Build history of the part. All positions in model axes, mm. A direction names the side the tool comes from. Round coordinates to 2 decimals unless told otherwise and drop trailing zeros. Write each loop counter-clockwise with the first axis right and the second up, starting at its lowest first coordinate (ties: lowest second). Pieces come first, ordered by that corner, then holes. Notation, with made-up numbers: (-24.5, 21.25) - (-7.5, 21.25) arc R6 cw to (-7.5, 30.25) - close; hole circle Ø4 at (84.25, -16.5). An arc over 180 degrees is marked (long way). One line per question, with ' | ' between items.
from build123d import *

# Parameters (mm, degrees)
F1_DEPTH = 50.8
F3_DEPTH = 25.4
F5_DEPTH = 12.7
F6_DEPTH = 12.7
F8_DEPTH = 25.401
F4_R     = 12.7
F9_DEPTH = 25.401


with BuildPart() as f1:
    # F0 (on Front) → F1 (new body)
    with BuildSketch(Plane.XZ):
        Polygon((-36.9852854972, 36.8870242119), (-62.3852854972, 36.8870242119), (-62.3852854972, -64.7129757881), (64.6147145028, -64.7129757881), (64.6147145028, -39.3129757881), (-36.9852854972, -39.3129757881), align=None)
    extrude(amount=F1_DEPTH)

    # F2 (on face) → F3 (cut)
    with BuildSketch(Plane.XY.offset(-39.3129757881)):
        with BuildLine():
            ThreePointArc((64.6147145028, -25.4), (57.1752267449, -43.3605122421), (39.2147145028, -50.8))
            Line((39.2147145028, -50.8), (64.6147145028, -50.8))
            Line((64.6147145028, -50.8), (64.6147145028, -25.4))
        make_face()
        with BuildLine():
            ThreePointArc((39.2147145028, 0), (57.1752267449, -7.4394877579), (64.6147145028, -25.4))
            Line((64.6147145028, -25.4), (64.6147145028, 0))
            Line((64.6147145028, 0), (39.2147145028, 0))
        make_face()
    extrude(amount=-F3_DEPTH, mode=Mode.SUBTRACT)

    # F5 (add): a face of the model
    f5_faces = [f1.faces().sort_by_distance(p)[0] for p in [
        (-36.9852854972, -25.4, -1.2129757881),
    ]]
    extrude(f5_faces, amount=F5_DEPTH)

    # F6 (cut): a face of the model
    f6_faces = [f1.faces().sort_by_distance(p)[0] for p in [
        (-62.3852854972, -25.4, -13.9129757881),
    ]]
    extrude(f6_faces, amount=-F6_DEPTH, mode=Mode.SUBTRACT)

    # F7 (on face) → F8 (cut, through all)
    with BuildSketch(Plane.YZ.offset(-24.2852854972)):
        with BuildLine():
            Line((-38.1, 36.8870242119), (-38.1, 11.4870242119))
            ThreePointArc((-38.1, 11.4870242119), (-25.4, -1.2129757881), (-12.7, 11.4870242119))
            Line((-12.7, 11.4870242119), (-12.7, 36.8870242119))
            Line((-12.7, 36.8870242119), (-38.1, 36.8870242119))
        make_face()
    extrude(amount=-F8_DEPTH, mode=Mode.SUBTRACT)

    # F4 (on face) → F9 (cut, through all)
    with BuildSketch(Plane.XY.offset(-39.3129757881)):
        with Locations((1.1147145028, -25.4)):
            Circle(F4_R)
        with Locations((39.2147145028, -25.4)):
            Circle(F4_R)
    extrude(amount=-F9_DEPTH, mode=Mode.SUBTRACT)


solid = f1.part
Q1. Pull direction Y, two halves, no side cores. Call faces 1 (the cylindrical face through (-36.81, -25.68, -1.21)), 2 (the flat face through (21, -25, -39.313)), 3 (the flat face through (-26, 0, -26)), 4 (the flat face through (-26, -50.8, -26)): +Y half, -Y half, draft (parallel to the pull), parting line (faces both ways), or undercut.
Found:
face 1: undercut | face 2: draft | face 3: +Y half | face 4: -Y half
Q2. Drill centre lines: L1, parallel to Y at x = -32, z = 12.5; L2, parallel to Z at x = -8.5, y = -9.5; L3, parallel to X at y = -7, z = 28.5. Where is each one in solid material? Low to high. Write a range as from..to.
Found:
L1: -50.8..-38.1, -12.7..0 | L2: -64.71..-39.31 | L3: -49.69..-24.29
Q3. Saw through at C-C, the plane z = -56.5. List the corners of the cut face in (x, y), then the cut area to 3 significant figures.
Found:
outline: (-49.69, -50.8) - (39.21, -50.8) arc R25.4 ccw to (39.21, 0) - (-49.69, 0) - close; hole circle Ø25.4 at (1.11, -25.4); hole circle Ø25.4 at (39.21, -25.4) | area: 4,520 mm^2
Q4. Drop flat-ended pins along their axis: pin 1 (4 mm diameter, centred on y = -11.5, z = 3.5, fed in from +X); pin 2 (7.5 mm diameter, centred on x = -33, z = 29, fed in from +Y). Give the stop position or say it passes through.
Found:
pin 1: x = -24.29 | pin 2: y = 0
Q5. Saw through at B-B, the plane x = 37.5. List the corners of the cut face in (y, z), then the cut area to 3 significant figures.
Found:
outline: (-50.8, -64.71) - (-37.98, -64.71) - (-37.98, -39.31) - (-50.8, -39.31) - close; (-12.82, -64.71) - (0, -64.71) - (0, -39.31) - (-12.82, -39.31) - close | area: 651 mm^2
Q6. Saw through at D-D, the plane y = -41.5. List the corners of the cut face in (x, z), then the cut area to 3 significant figures.
Found:
outline: (-49.69, -64.71) - (58.86, -64.71) - (58.86, -39.31) - (-24.29, -39.31) - (-24.29, 36.89) - (-49.69, 36.89) - close | area: 4,690 mm^2
Q7. Which spindle directions (+Z, -Z, +X, -X, +Y, -Y) get a long thin tool onto all of the face, cutting with end or side? Do faces 5 (the flat face through (-24.285, -25, -10)), 6 (the flat face through (-37, -38.1, 24)), 7 (the flat face through (-37, -44, 36.887)). Say none if no direction does.
Found:
face 5: +Z, +X, +Y, -Y | face 6: +Z, +X, -X | face 7: +Z, +X, -X, +Y, -Y
Q8. Saw through at A-A, the plane z = 31. List the corners of the cut face in (x, y).
Found:
outline: (-49.69, -50.8) - (-24.29, -50.8) - (-24.29, -38.1) - (-49.69, -38.1) - close; (-49.69, -12.7) - (-24.29, -12.7) - (-24.29, 0) - (-49.69, 0) - close
